from build123d import *

# Parameters (mm, degrees)
SKETCH_1_R      = 1
EXTRUDE_1_DEPTH = 3


with BuildPart() as part:
    # 草图1 → 凸台-拉伸1 (new body)
    with BuildSketch(Plane.XY):
        with BuildLine():
            Line((-374.926675411, 73.771047931), (-374.926675411, 85.377996683))
            ThreePointArc((-374.926675411, 85.377996683), (-374.833212563, 86.742006081), (-374.554571083, 88.080518639))
            ThreePointArc((-374.554571083, 88.080518639), (-378.521236494, 94.132867012), (-383.975961006, 89.377729178))
            Line((-383.975961006, 89.377729178), (-383.975961006, 52.22545565))
            Line((-383.975961006, 52.22545565), (-383.975961006, 37.377729178))
            ThreePointArc((-383.975961006, 37.377729178), (-379.175961006, 32.577729178), (-374.375961006, 37.377729178))
            Line((-374.375961006, 37.377729178), (-374.375961006, 62.224119392))
            ThreePointArc((-374.375961006, 62.224119392), (-374.18461917, 63.077791251), (-373.647205362, 63.76811997))
            ThreePointArc((-373.647205362, 63.76811997), (-371.745473945, 68.072262412), (-374.066514555, 72.165548992))
            ThreePointArc((-374.066514555, 72.165548992), (-374.68996635, 72.864697969), (-374.926675411, 73.771047931))
        make_face()
        with Locations((-379.175961006, 79.377729178)):
            Circle(SKETCH_1_R, mode=Mode.SUBTRACT)
        with BuildLine():
            Line((-382.175961006, 89.377729178), (-382.175961006, 52.97993897))
            ThreePointArc((-382.175961006, 52.97993897), (-381.575961006, 52.37993897), (-380.975961006, 52.97993897))
            Line((-380.975961006, 52.97993897), (-380.975961006, 85.964352253))
            ThreePointArc((-380.975961006, 85.964352253), (-380.724426098, 86.459873764), (-380.175961006, 86.549302053))
            ThreePointArc((-380.175961006, 86.549302053), (-376.726471263, 91.109779986), (-382.175961006, 89.377729178))
        make_face(mode=Mode.SUBTRACT)
        with BuildLine():
            Line((-378.775961006, 42.811088271), (-378.775961006, 64.56147291))
            ThreePointArc((-378.775961006, 64.56147291), (-378.556266961, 64.975512245), (-378.09024672, 65.025703676))
            ThreePointArc((-378.09024672, 65.025703676), (-374.491724992, 69.492924003), (-379.975961006, 67.811088271))
            Line((-379.975961006, 67.811088271), (-379.975961006, 42.811088271))
            ThreePointArc((-379.975961006, 42.811088271), (-379.375961006, 42.211088271), (-378.775961006, 42.811088271))
        make_face(mode=Mode.SUBTRACT)
        with BuildLine():
            Line((-376.175961006, 37.377729178), (-376.175961006, 62.377729178))
            ThreePointArc((-376.175961006, 62.377729178), (-376.775961006, 62.977729178), (-377.375961006, 62.377729178))
            Line((-377.375961006, 62.377729178), (-377.375961006, 40.62734454))
            ThreePointArc((-377.375961006, 40.62734454), (-377.59565505, 40.213305204), (-378.061675291, 40.163113774))
            ThreePointArc((-378.061675291, 40.163113774), (-381.660197019, 35.695893446), (-376.175961006, 37.377729178))
        make_face(mode=Mode.SUBTRACT)
    extrude(amount=EXTRUDE_1_DEPTH)


solid = part.part
Can you work these out from the model? Positions are in its coordinate system, mm. A direction names the side the tool comes from. Round coordinates to 2 decimals unless told otherwise and drop trailing zeros. Loops run counter-clockwise (first coordinate to the right, second up) from the corner with the lowest first, then second, coordinate; pieces in that order, holes last. Notation, with made-up numbers: (89.25, 35.25) - (142.25, 35.25) arc R34 cw to (142.25, 67.25) - close; hole circle Ø11 at (26, -38.75). An arc over 180 degrees is marked (long way). Use CSV: the item, a comma, the result in double quotes. Start each with the question number.
1) If we section it at B-B on x = -381.5: Write out the boundary of the cut face in (y, z).
2) If we section it at C-C on y = 66.5: Write out the boundary of the cut face in (x, z), plus the area to 3 significant figures.
3) We'd pull the mould along X, two halves only. Please class faces 4 (the cylindrical face through (-374.43, 69.4, 1.48)), 5 (the cylindrical face through (-371.743, 68.004, 1.479)), 6 (the flat face through (-378, 64, 0)): released by +X, released by -X, zero draft, split by the parting line, or undercut.
4) If we section it at A-A on y = 74.5: Write out the boundary of the cut face in (x, z), plus the area to 3 significant figures.
5) Please list where these lines run through material, in increasing order: probe 1 along X at (y, z) = (50, 0.5); probe 2 along X at (y, z) = (58.5, 1.35); probe 3 along Y at (x, z) = (-381.5, 0.3). Write a range as [from, to].
6) For faces 1 (the flat face through (-374.376, 50, 1)), 2 (the flat face through (-380.976, 69, 1)), 3 (the cylindrical face through (-374.68, 72.85, 1.48)), which set-ups out of +Z, -Z, +X, -X, +Y, -Y let a thin tool reach every point of the face, with its end or its side?
7) For pin 1 Ø1 at (x, z) = (-374.5, 1) entering from +Y; pin 2 Ø0.9 at (y, z) = (80, 2) entering from +X; pin 3 Ø1.8 at (x, y) = (-379.18, 79.38) entering from +Z; pin 4 Ø1.5 at (y, z) = (65, 2) entering from +X, each with a flat end and sliding along its axis, tell me the tip position at first contact or that it passes through.
8) If we section it at D-D on z = 1.45: Write out the boundary of the cut face in (x, y).
Geometry results:
1,outline,"(33.18, 0) - (35.48, 0) - (35.48, 3) - (33.18, 3) - close; (39.27, 0) - (52.38, 0) - (52.38, 3) - (39.27, 3) - close; (91.27, 0) - (93.58, 0) - (93.58, 3) - (91.27, 3) - close"
2,outline,"(-383.98, 0) - (-382.18, 0) - (-382.18, 3) - (-383.98, 3) - close; (-380.98, 0) - (-379.98, 0) - (-379.98, 3) - (-380.98, 3) - close; (-374.28, 0) - (-371.91, 0) - (-371.91, 3) - (-374.28, 3) - close"
2,area,"15.5 mm2"
3,face 4,"undercut"
3,face 5,"released by +X"
3,face 6,"zero draft"
4,outline,"(-383.98, 0) - (-382.18, 0) - (-382.18, 3) - (-383.98, 3) - close; (-380.98, 0) - (-374.93, 0) - (-374.93, 3) - (-380.98, 3) - close"
4,area,"23.5 mm2"
5,probe 1,"x = [-383.98, -379.98], [-378.78, -377.38], [-376.18, -374.38]"
5,probe 2,"x = [-383.98, -382.18], [-380.98, -379.98], [-378.78, -377.38], [-376.18, -374.38]"
5,probe 3,"y = [33.18, 35.48], [39.27, 52.38], [91.27, 93.58]"
6,face 1,"+Z, -Z, +X, -Y"
6,face 2,"+Z, -Z"
6,face 3,"+Z, -Z, +X"
7,pin 1,"stops at y = 91.74"
7,pin 2,"stops at x = -374.93"
7,pin 3,"passes through"
7,pin 4,"stops at x = -372.16"
8,outline,"(-383.98, 37.38) arc R4.8 ccw to (-374.38, 37.38) - (-374.38, 62.22) arc R2 cw to (-373.65, 63.77) arc R5.24 ccw to (-374.07, 72.17) arc R2 cw to (-374.93, 73.77) - (-374.93, 85.38) arc R10 cw to (-374.55, 88.08) arc R4.8 ccw (long way) to (-383.98, 89.38) - close; hole (-382.18, 52.98) arc R0.6 ccw to (-380.98, 52.98) - (-380.98, 85.96) arc R0.61 cw to (-380.18, 86.55) arc R3 ccw (long way) to (-382.18, 89.38) - close; hole circle Ø2 at (-379.18, 79.38); hole (-379.98, 42.81) arc R0.6 ccw to (-378.78, 42.81) - (-378.78, 64.56) arc R0.5 cw to (-378.09, 65.03) arc R3 ccw (long way) to (-379.98, 67.81) - close; hole (-378.06, 40.16) arc R3 ccw (long way) to (-376.18, 37.38) - (-376.18, 62.38) arc R0.6 ccw to (-377.38, 62.38) - (-377.38, 40.63) arc R0.5 cw to start"
